Build history of the part. All positions in model axes, mm. Give positions to 0.01 mm unless a question says otherwise; leave off trailing zeros. Write each loop counter-clockwise with the first axis right and the second up, starting at its lowest first coordinate (ties: lowest second). Pieces come first, ordered by that corner, then holes.
Autodesk Inventor part; units mm, degrees
ref_plane "YZ Plane" through (0, 0, 0) normal (1, 0, 0) x (0, 1, 0)
ref_plane "XZ Plane" through (0, 0, 0) normal (0, 1, 0) x (-1, 0, 0)
ref_plane "XY Plane" through (0, 0, 0) normal (0, 0, 1) x (1, 0, 0)
sketch "Sketch1" plane through (0, 0, 0) normal (0, 1, 0) x (-1, 0, 0)
  line L0 (62.5322, -45.6018) -> (-188.8149, -45.6018) construction
  arc A0 (-158.4408, -29.8487) -> (-158.4408, -61.3549) centre (-155.6408, -45.6018) ccw
  arc A1 (-8.8908, -67.4293) -> (-8.8908, -23.7744) centre (-11.6408, -45.6018) ccw
  line L1 (-8.8908, -67.4293) -> (-71.8908, -75.3665)
  line L2 (-8.8908, -23.7744) -> (-71.8908, -15.8371)
  line L3 (-80.8908, -75.1389) -> (-158.4408, -61.3549)
  line L4 (-158.4408, -29.8487) -> (-80.8908, -16.0647)
  arc A2 (-80.8908, -75.1389) -> (-71.8908, -75.3665) centre (-75.6408, -45.6018) ccw
  arc A3 (-71.8908, -15.8371) -> (-80.8908, -16.0647) centre (-75.6408, -45.6018) ccw
  circle A4 centre (-155.6408, -45.6018) radius 7
  circle A5 centre (-75.6408, -45.6018) radius 7
  circle A6 centre (-37.5408, -45.6018) radius 12 construction
  circle A7 centre (-25.5408, -45.6018) radius 2
  circle A8 centre (-37.5408, -33.6018) radius 2
  circle A9 centre (-49.5408, -45.6018) radius 2
  circle A10 centre (-37.5408, -57.6018) radius 2
  circle A11 centre (-75.6408, -45.6018) radius 38.1 construction
  circle A12 centre (-155.6408, -45.6018) radius 38.1 construction
  circle A13 centre (-37.5408, -45.6018) radius 5
  circle A14 centre (-11.6408, -45.6018) radius 16 construction
  circle A15 centre (-25.5408, -63.6018) radius 2
  circle A16 centre (-25.5408, -27.6018) radius 2
  circle A17 centre (-115.6408, -57.6018) radius 2
  circle A18 centre (-115.6408, -33.6018) radius 2
  point P0 (0, 0)
  dimension "d9" = 24
  dimension "d16" = 76.2
  dimension "d0" = 32
  dimension "d1" = 44
  dimension "d3" = 80
  dimension "d4" = 64
  dimension "d5" = 14
  dimension "d6" = 14
  dimension "d7" = 30
  dimension "d8" = 30
  dimension "d10" = 4
  dimension "d13" = 360
  dimension "d15" = 12
  dimension "d17" = 76.2
  dimension "d18" = 10
  dimension "d19" = 32
  dimension "d20" = 4
  dimension "d21" = 4
  dimension "d22" = 4
  dimension "d23" = 4
  dimension "d24" = 40
  dimension "d25" = 40
  dimension "d26" = 12
  dimension "d27" = 12
  dimension "d30" = 36
  dimension "d31" = 18
extrude "Extrusion1" add sketch "Sketch1" along normal blind 3.175
properties part number "bottombeanv2"
1. Saw through at A-A on x = 79. Give the cut face in (y, z) (3 decimals), plus the area to 3 significant figures.
2. Drop flat-ended pins along their axis: pin 1 (1.5 mm diameter, centred on x = 28.5, y = 0.5, fed in from -Z); pin 2 (1 mm diameter, centred on x = 105.5, y = 2.5, fed in from -Z). Give the stop position or say it passes through.
3. Saw through at C-C on x = 153.5. Give the cut face in (y, z) (1 decimal), plus the area to 3 significant figures.
4. Drill centre lines: line 1 along X through (y, z) = (1.2, -32.5); line 2 along X through (y, z) = (0.2, -34.5); line 3 along X through (y, z) = (2.7, -41.5). Where is each one in solid material? Low to high.
5. Mould opens along Z. For faces 1 (the face through (171.638, 1.565, -45.914)), 2 (the face through (82, 0, -52)), 3 (the face through (113.79, 1.57, -56.84)) say: pulls with the +Z half, pulls with the -Z half, needs draft (parallel to the pull), parting line crosses it, or undercut.
6. Saw through at B-B on y = 0.6. Count the separate pieces of the cut face and the enclosed holes in it, plus the area to 3 significant figures.
7. Saw through at D-D on x = 109. Give the cut face in (y, z) (3 decimals), plus the area to 3 significant figures.
Outcome:
1. outline: (0, -75.413) - (3.175, -75.413) - (3.175, -51.743) - (0, -51.743) - close; (0, -39.46) - (3.175, -39.46) - (3.175, -15.79) - (0, -15.79) - close
1. area: 150 mm2
2. pin 1: stops at z = -69.99
2. pin 2: stops at z = -70.85
3. outline: (0, -62.2) - (3.2, -62.2) - (3.2, -52.3) - (0, -52.3) - close; (0, -38.9) - (3.2, -38.9) - (3.2, -29) - (0, -29) - close
3. area: 63.3 mm2
4. line 1: x = -6.03 to 35.87, 39.21 to 113.97, 117.31 to 164.82
4. line 2: x = -7.35 to 35.75, 39.33 to 113.85, 117.43 to 167.16
4. line 3: x = -9.97 to 34.68, 40.4 to 69.97, 81.31 to 149.97, 161.31 to 171.11
5. face 1: parting line crosses it
5. face 2: needs draft
5. face 3: undercut
6. separate pieces: 1
6. enclosed holes: 11
6. area: 7,770 mm2
7. outline: (0, -70.143) - (3.175, -70.143) - (3.175, -21.061) - (0, -21.061) - close
7. area: 156 mm2
